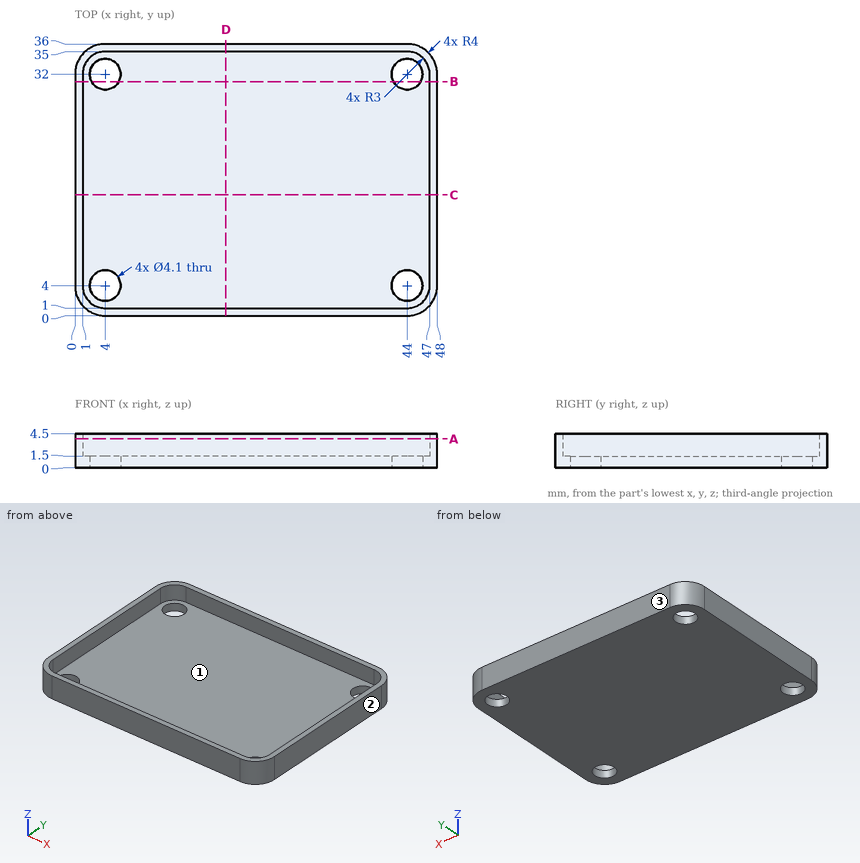
Answer from the drawing. Dimensions are ordinates in mm from the lowest x, y and z of the part. Give positions to 0.01 mm unless a question says otherwise; leave off trailing zeros. Order: outer loops, then holes, each group sorted by start corner. A loop starts at its lowest first (then second) coordinate and runs counter-clockwise, first axis right, second up.
(1) Straight lines are drawn through the part: L1, parallel to X at y = 32, z = 0.65; L2, parallel to Y at x = 44, z = 0.7; L3, parallel to Y at x = 41, z = 3.95. For each, find the intervals that lie inside material, in ascending order.
(2) Find section A-A (z = 3.8). Give the vertices of the cut face in (x, y).
(3) Given pin 1 (10 mm diameter, centred on x = 28.5, y = 10, fed in from +Z), flat-ended and moving along its own axis, determine where the tip first touches the part or whether it passes through.
(4) Find section D-D (x = 20). Give the vertices of the cut face in (y, z).
(5) For a pull along Y with two mould halves and no side action, classify the marked faces 1, 2 and 3 as released by +Y, released by -Y, zero draft, split by the parting line, or undercut.
(6) Find section B-B (y = 31). Give the vertices of the cut face in (x, z), plus the area to 3 significant figures.
(7) Find section C-C (y = 16). Give the vertices of the cut face in (x, z).
Result sheet:
1. L1: x = 0 to 1.95, 6.05 to 41.95, 46.05 to 48
1. L2: y = 0 to 1.95, 6.05 to 29.95, 34.05 to 36
1. L3: y = 0 to 1, 35 to 36
2. outline: (0, 4) arc R4 ccw to (4, 0) - (44, 0) arc R4 ccw to (48, 4) - (48, 32) arc R4 ccw to (44, 36) - (4, 36) arc R4 ccw to (0, 32) - close; hole (1, 4) arc R3 ccw to (4, 1) - (44, 1) arc R3 ccw to (47, 4) - (47, 32) arc R3 ccw to (44, 35) - (4, 35) arc R3 ccw to (1, 32) - close
3. pin 1: stops at z = 1.5
4. outline: (0, 0) - (36, 0) - (36, 4.5) - (35, 4.5) - (35, 1.5) - (1, 1.5) - (1, 4.5) - (0, 4.5) - close
5. face 1: undercut
5. face 2: zero draft
5. face 3: released by +Y
6. outline: (0, 0) - (2.21, 0) - (2.21, 1.5) - (1, 1.5) - (1, 4.5) - (0, 4.5) - close; (5.79, 0) - (42.21, 0) - (42.21, 1.5) - (5.79, 1.5) - close; (45.79, 0) - (48, 0) - (48, 4.5) - (47, 4.5) - (47, 1.5) - (45.79, 1.5) - close
6. area: 67.3 mm2
7. outline: (0, 0) - (48, 0) - (48, 4.5) - (47, 4.5) - (47, 1.5) - (1, 1.5) - (1, 4.5) - (0, 4.5) - close
